```python
from build123d import *

# Parameters (mm, degrees)
ESQUISSE1_R        = 2
BOSS_EXTRU_1_DEPTH = 5
CONG_1_R           = 5


with BuildPart() as part:
    # Esquisse1 → Boss.-Extru.1 (new body)
    with BuildSketch(Plane(origin=(0, 0, 0), x_dir=(1, 0, 0), z_dir=(0, 1, 0))):
        with BuildLine():
            Line((0, 10.29493472), (0, 3.789721085))
            Line((0, 3.789721085), (10, 0))
            Line((10, 0), (40, 0))
            Line((40, 0), (67.189233611, -12.678547852))
            ThreePointArc((67.189233611, -12.678547852), (72.504937806, -10.743789751), (70.570179705, -5.428085556))
            Line((70.570179705, -5.428085556), (41.421148718, 8.164330821))
            ThreePointArc((41.421148718, 8.164330821), (39.877944642, 7.977690672), (38.669460337, 7))
            Line((38.669460337, 7), (13.843067102, 7))
            Line((13.843067102, 7), (5.148668105, 10.29493472))
            Line((5.148668105, 10.29493472), (0, 10.29493472))
        make_face()
        with Locations(Location((68.879706658, -9.053316704, 0), (0, 0, 270))):
            Circle(ESQUISSE1_R, mode=Mode.SUBTRACT)
        with Locations(Location((41.690473047, 3.625231148, 0), (0, 0, 270))):
            Circle(ESQUISSE1_R, mode=Mode.SUBTRACT)
    extrude(amount=BOSS_EXTRU_1_DEPTH)

    # Congé1
    cong_1_edges = [part.edges().sort_by_distance(p)[0] for p in [
        (13.843067102, 2.5, -7),
        (38.669460337, 2.5, -7),
        (40, 2.5, 0),
        (10, 2.5, 0),
        (0, 2.5, -3.789721085),
    ]]
    fillet(cong_1_edges, radius=CONG_1_R)


solid = part.part
```
Build history of the part. All positions in model axes, mm. A direction names the side the tool comes from. Coordinates: 2 decimals unless noted, no trailing zeros. Order: outer loops, then holes, each group sorted by start corner. A loop starts at its lowest first (then second) coordinate and runs counter-clockwise, first axis right, second up. Notation, with made-up numbers: (62, 87.5) -> (120, 87.5) arc R24 cw to (120, 97.5) -> close; hole circle Ø6 at (27.5, -23.5). An arc over 180 degrees is marked (long way). Answer in a Markdown table with one row per item. Add a question column.
Q1. Mould opens along Z. For faces 1 (the face through (36, 0, -2)), 2 (the face through (39.916, 2.465, -2.702)), 3 (the face through (3, 2, -10.295)) say: +Z half, -Z half, draft (parallel to the pull), parting line (faces both ways), or undercut.
Q2. Band-saw the part on C-C, the plane x = 25. List the corners of the cut face in (y, z).
Q3. Which spindle directions (+Z, -Z, +X, -X, +Y, -Y) get a long thin tool onto all of the face, cutting with end or side? Do faces 4 (the face through (13.846, 2.535, -7.084)), 5 (the face through (36, 5, -2)), 6 (the face through (25, 2, 0)). Say none if no direction does.
Q4. Band-saw the part on A-A, the plane y = 1.75. List the corners of the cut face in (x, z), then the cut area to 3 significant figures.
Q5. Band-saw the part on B-B, the plane z = -4. List the corners of the cut face in (x, y), then the cut area to 3 significant figures.
Q6. Drop flat-ended pins along their axis: pin 1 (1 mm diameter, centred on y = 1, z = 5.5, fed in from -X); pin 2 (1.5 mm diameter, centred on x = 25, y = 3.5, fed in from -Z); pin 3 (2 mm diameter, centred on x = 29, y = 1.5, fed in from +Z). Give the stop position or say it passes through.
Q7. Band-saw the part on D-D, the plane z = 1.5. List the corners of the cut face in (x, y).
Q8. Wall check: line 1 along Z through (x, y) = (18, 3.9); line 2 along X through (y, z) = (4.4, -4.5); line 3 along X through (y, z) = (1.7, 9.5). Give the ranges that are in metal, low to high. Write a range as [from, to].
Answers follow:
| question | item | result |
|---|---|---|
| 1 | face 1 | draft |
| 1 | face 2 | undercut |
| 1 | face 3 | -Z half |
| 2 | outline | (0, -7) -> (5, -7) -> (5, 0) -> (0, 0) -> close |
| 3 | face 4 | -Z, +Y, -Y |
| 3 | face 5 | +Z, -Z, +X, -X, +Y |
| 3 | face 6 | +Z, -X, +Y, -Y |
| 4 | outline | (0, -10.29) -> (5.15, -10.29) -> (12.99, -7.32) arc R5 cw to (14.76, -7) -> (36.81, -7) arc R5 cw to (39.48, -7.77) arc R2.81 ccw to (41.42, -8.16) -> (70.57, 5.43) arc R4 ccw to (67.19, 12.68) -> (41, 0.47) arc R5 cw to (38.89, 0) -> (10.92, 0) arc R5 ccw to (9.14, -0.32) -> (3.23, -2.57) arc R5 ccw to (0, -7.24) -> close; hole circle Ø4 at (41.69, -3.63); hole circle Ø4 at (68.88, 9.05) |
| 4 | area | 546 mm^2 |
| 5 | outline | (1.19, 0) -> (39.73, 0) -> (39.73, 5) -> (1.19, 5) -> close; (43.66, 0) -> (50.35, 0) -> (50.35, 5) -> (43.66, 5) -> close |
| 5 | area | 226 mm^2 |
| 6 | pin 1 | x = 50.72 |
| 6 | pin 2 | z = -7 |
| 6 | pin 3 | z = 0 |
| 7 | outline | (43.22, 0) -> (62.15, 0) -> (62.15, 5) -> (43.22, 5) -> close |
| 8 | line 1 | [-7, 0] |
| 8 | line 2 | [0.82, 39.89], [43.49, 49.28] |
| 8 | line 3 | [60.37, 66.93], [70.83, 72.85] |
